Design review of the part built by this model. Coordinates are the model's own, in mm. Face numbers are marked on the shaded views. A direction names the side the tool comes from. Coordinates: 2 decimals unless noted, no trailing zeros. Loops run counter-clockwise (first coordinate to the right, second up) from the corner with the lowest first, then second, coordinate; pieces in that order, holes last. Notation, with made-up numbers: (-37.75, 16) - (-3.75, 16) arc R20 ccw to (-3.75, 20) - close; hole circle Ø9 at (-24.75, 30). An arc over 180 degrees is marked (long way). Return JSON: item names as keys, results as strings. Group by question number.
Autodesk Inventor part; units mm, degrees
ref_plane "YZ Plane" through (0, 0, 0) normal (1, 0, 0) x (0, 1, 0)
ref_plane "XZ Plane" through (0, 0, 0) normal (0, 1, 0) x (-1, 0, 0)
ref_plane "XY Plane" through (0, 0, 0) normal (0, 0, 1) x (1, 0, 0)
sketch "Sketch1" plane through (0, 0, 0) normal (0, 0, 1) x (1, 0, 0)
  circle A0 centre (0, 0) radius 6
  circle A1 centre (0, 0) radius 2
  dimension "d0" = 12
  dimension "d1" = 4
extrude "Extrusion1" add sketch "Sketch1" along normal blind 10
sketch "Sketch3" plane through (0, 0, 10) normal (0, 0, 1) x (1, 0, 0)
  line L0 (0, 0) -> (25, 0) construction
  arc A0 (9.6912, 0.8) -> (5.6912, 1.9) centre (3.7521, -12.9741) ccw
  circle A1 centre (0, 0) radius 6
  arc A2 (9.6912, -0.8) -> (9.6912, 0.8) centre (-10.2928, 0) ccw
  arc A3 (5.6912, -1.9) -> (9.6912, -0.8) centre (3.7521, 12.9741) ccw
  arc A4 (5.6912, -1.9) -> (5.6912, 1.9) centre (0, 0) ccw
  arc A5 (6.9097, 6.8422) -> (3.1384, 5.1137) centre (11.2139, -7.527) ccw
  arc A6 (7.9381, 5.6166) -> (6.9097, 6.8422) centre (-7.8847, -6.6161) ccw
  arc A7 (5.581, 2.2028) -> (7.9381, 5.6166) centre (-5.4653, 12.3506) ccw
  arc A8 (5.581, 2.2028) -> (3.1384, 5.1137) centre (0, 0) ccw
  arc A9 (0.895, 9.6829) -> (-0.8829, 5.9347) centre (13.4286, 1.4421) ccw
  arc A10 (2.4707, 9.4051) -> (0.895, 9.6829) centre (-1.7873, -10.1364) ccw
  arc A11 (2.8594, 5.2748) -> (2.4707, 9.4051) centre (-12.1255, 5.948) ccw
  arc A12 (2.8594, 5.2748) -> (-0.8829, 5.9347) centre (0, 0) ccw
  arc A13 (-5.5384, 7.9928) -> (-4.4911, 3.9787) centre (9.3599, 9.7365) ccw
  arc A14 (-4.1528, 8.7928) -> (-5.5384, 7.9928) centre (5.1464, -8.9138) ccw
  arc A15 (-1.2002, 5.8787) -> (-4.1528, 8.7928) centre (-13.112, -3.2377) ccw
  arc A16 (-1.2002, 5.8787) -> (-4.4911, 3.9787) centre (0, 0) ccw
  arc A17 (-9.3804, 2.5628) -> (-5.9978, 0.1611) centre (0.9116, 13.475) ccw
  arc A18 (-8.8332, 4.0663) -> (-9.3804, 2.5628) centre (9.672, -3.5203) ccw
  arc A19 (-4.6982, 3.7319) -> (-8.8332, 4.0663) centre (-7.9632, -10.9084) ccw
  arc A20 (-4.6982, 3.7319) -> (-5.9978, 0.1611) centre (0, 0) ccw
  arc A21 (-8.8332, -4.0663) -> (-4.6982, -3.7319) centre (-7.9632, 10.9084) ccw
  arc A22 (-9.3804, -2.5628) -> (-8.8332, -4.0663) centre (9.672, 3.5203) ccw
  arc A23 (-5.9978, -0.1611) -> (-9.3804, -2.5628) centre (0.9116, -13.475) ccw
  arc A24 (-5.9978, -0.1611) -> (-4.6982, -3.7319) centre (0, 0) ccw
  arc A25 (-4.1528, -8.7928) -> (-1.2002, -5.8787) centre (-13.112, 3.2377) ccw
  arc A26 (-5.5384, -7.9928) -> (-4.1528, -8.7928) centre (5.1464, 8.9138) ccw
  arc A27 (-4.4911, -3.9787) -> (-5.5384, -7.9928) centre (9.3599, -9.7365) ccw
  arc A28 (-4.4911, -3.9787) -> (-1.2002, -5.8787) centre (0, 0) ccw
  arc A29 (2.4707, -9.4051) -> (2.8594, -5.2748) centre (-12.1255, -5.948) ccw
  arc A30 (0.895, -9.6829) -> (2.4707, -9.4051) centre (-1.7873, 10.1364) ccw
  arc A31 (-0.8829, -5.9347) -> (0.895, -9.6829) centre (13.4286, -1.4421) ccw
  arc A32 (-0.8829, -5.9347) -> (2.8594, -5.2748) centre (0, 0) ccw
  arc A33 (7.9381, -5.6166) -> (5.581, -2.2028) centre (-5.4653, -12.3506) ccw
  arc A34 (6.9097, -6.8422) -> (7.9381, -5.6166) centre (-7.8847, 6.6161) ccw
  arc A35 (3.1384, -5.1137) -> (6.9097, -6.8422) centre (11.2139, 7.527) ccw
  arc A36 (3.1384, -5.1137) -> (5.581, -2.2028) centre (0, 0) ccw
  point P0 (9.7072, 0)
  point P1 (7.4362, 6.2397)
  point P2 (1.6856, 9.5598)
  point P3 (-4.8536, 8.4067)
  point P4 (-9.1218, 3.3201)
  point P5 (-9.1218, -3.3201)
  point P6 (-4.8536, -8.4067)
  point P7 (1.6856, -9.5598)
  point P8 (7.4362, -6.2397)
  dimension "d8" = 25
  dimension "d9" = 15
  dimension "d10" = 1.6
  dimension "d11" = 20
  dimension "d12" = 4
  dimension "d13" = 1.1
  dimension "d14" = 15
  dimension "d15" = 1.1
  dimension "d16" = 4
  dimension "d19" = 360
extrude "Extrusion3" add sketch "Sketch3" against normal blind 10 contours A2 A3 A1 A0 | A1 A5 A6 A7 | A33 A34 A35 A1 | A1 A9 A10 A11 | A29 A30 A31 A1 | A1 A13 A14 A15 | A25 A26 A27 A1 | A1 A17 A18 A19 | A21 A22 A23 A1
properties part number "GA002" material "ABS Plastic"
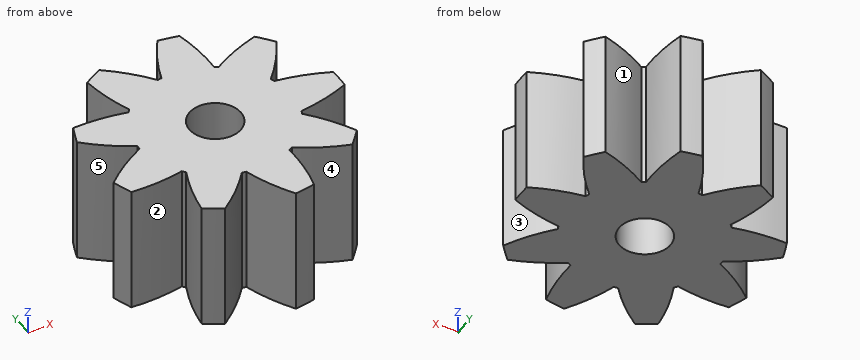
Item 1: For P1, Ø2, axis at x = -4.5, z = 7.5, coming from the -Y side; P2, Ø3.5, axis at x = 0, y = 0, coming from the -Z side; P3, Ø6, axis at x = 4.5, z = 1.5, coming from the -Y side; P4, Ø3, axis at y = 6.5, z = 8.5, coming from the -X side, all flat-tipped, find the tip position at first contact; note any pin that passes through.
Item 2: For the marked faces 1, 2, 3, 4 and 5, list the 3-axis set-ups (+Z, -Z, +X, -X, +Y, -Y) from which the entire face can be reached by the end or side of a thin tool; tool diameter is ignored.
Item 3: To check wall thickness, follow line 1 (X direction, y = -0.25, z = 8.75); line 2 (X direction, y = 7, z = 3); line 3 (Y direction, x = -6.5, z = 0.5). State the ranges of each line that lie inside material, in increasing order. Write a range as from..to.
Item 4: Add section B-B (x = -3.25). State the section outline as (y, z) points.
Item 5: Add section A-A (x = 0). State the section outline as (y, z) points.
Answers below:
{
 "1": {"P1": "stops at y = -8.79", "P2": "passes through", "P3": "stops at y = -9.59", "P4": "stops at x = -5.54"},
 "2": {"face 1": "+Z, -Z, +Y", "face 2": "+Z, -Z", "face 3": "+Z, -Z, +X", "face 4": "+Z, -Z, -Y", "face 5": "+Z, -Z, -X"},
 "3": {"line 1": "x = -6.17..-1.98, 1.98..9.71", "line 2": "x = -5.39..-2.15, -0.5..2.84", "line 3": "y = -4.02..-0.43, 0.43..4.02"},
 "4": {"outline": "(-8.06, 0) - (8.06, 0) - (8.06, 10) - (-8.06, 10) - close"},
 "5": {"outline": "(-8.13, 0) - (-2, 0) - (-2, 10) - (-8.13, 10) - close; (2, 0) - (8.13, 0) - (8.13, 10) - (2, 10) - close"}
}
